Here's how the part is built. I have some questions about the finished solid (model axes, mm). Face numbers are marked on the shaded views. A direction names the side the tool comes from. Coordinates: 2 decimals unless noted, no trailing zeros. Order: outer loops, then holes, each group sorted by start corner. A loop starts at its lowest first (then second) coordinate and runs counter-clockwise, first axis right, second up. Notation, with made-up numbers: (21, 39) - (28, 39) arc R32 ccw to (28, 67) - close; hole circle Ø8 at (-2.5, 13.5). An arc over 180 degrees is marked (long way). Answer as CSV lines item,"result". Start each with the question number.
Q1. I need wall thicknesses on line 1 (X direction, y = -12, z = 24.5); line 2 (X direction, y = 99, z = 22); line 3 (Y direction, x = -56, z = 25). Which ranges of each line are inside material? Lowest first, please.
Q2. Suppose I cut it at D-D (x = 5.5). Please give me the cut outline in (y, z).
Q3. For pin 1 Ø2 at (x, y) = (26, 102.5) entering from +Z; pin 2 Ø12.5 at (y, z) = (105.5, 34.5) entering from +X; pin 3 Ø7.5 at (x, z) = (46, 32) entering from +Y, each with a flat end and sliding along its axis, tell me the tip position at first contact or that it passes through.
Q4. For the marked faces 1, 2 and 3, which set-ups out of +Z, -Z, +X, -X, +Y, -Y let a thin tool reach every point of the face, with its end or its side?
Q5. Suppose I cut it at B-B (y = 43.5). Please give me the cut outline in (x, z).
Q6. Suppose I cut it at C-C (z = 21). Please give me the cut outline in (x, y).
Q7. Thinking about a two-plate mould opening in X: for the marked faces 4, 5 and 6, which applies, released by +X, released by -X, zero draft, split by the parting line, or undercut?
Q8. Suppose I cut it at A-A (z = 37). Please give me the cut outline in (x, y), then the cut area to 3 significant figures.
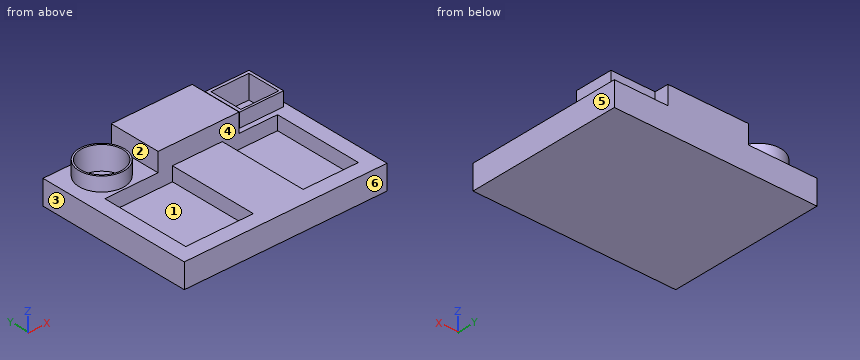
from build123d import *

# Parameters (mm, degrees)
F0_W      = 216
F0_H      = 166
F1_DEPTH  = 26
F2_W      = 184
F2_H      = 95
F3_DEPTH  = 15
F4_W      = 86.176178
F4_H      = 55
F5_DEPTH  = 20
F6_W      = 53.007906
F6_H      = 95
F7_DEPTH  = 15
F8_R      = 24.127346
F9_DEPTH  = 15
F10_R     = 22.341692
F11_DEPTH = 25
F12_W     = 46.807702
F12_H     = 40.58332
F13_DEPTH = 15
F14_W     = 40.349298
F14_H     = 35.074882
F15_DEPTH = 25


with BuildPart() as f1:
    # F0 (on Top) → F1 (new body)
    with BuildSketch(Plane.XY):
        with Locations((-35.592673, 44.704702)):
            Rectangle(F0_W, F0_H)
    extrude(amount=F1_DEPTH)

    # F2 (on face) → F3 (cut)
    with BuildSketch(Plane.XY.offset(26)):
        with Locations((-35.592673, 25.204702)):
            Rectangle(F2_W, F2_H)
    extrude(amount=-F3_DEPTH, mode=Mode.SUBTRACT)

    # F4 (on face) → F5 (join)
    with BuildSketch(Plane.XY.offset(26)):
        with Locations((-27.75256, 100.204702)):
            Rectangle(F4_W, F4_H)
    extrude(amount=F5_DEPTH)

    # F6 (on face) → F7 (join)
    with BuildSketch(Plane.XY.offset(11)):
        with Locations((-28.99965, 25.204702)):
            Rectangle(F6_W, F6_H)
    extrude(amount=F7_DEPTH)

    # F8 (on face) → F9 (join)
    with BuildSketch(Plane.XY.offset(26)):
        with Locations((-106.665462, 99.426791)):
            Circle(F8_R)
    extrude(amount=F9_DEPTH)

    # F10 (on face) → F11 (cut)
    with BuildSketch(Plane.XY.offset(41)):
        with Locations((-106.665462, 99.426791)):
            Circle(F10_R)
    extrude(amount=-F11_DEPTH, mode=Mode.SUBTRACT)

    # F12 (on face) → F13 (join)
    with BuildSketch(Plane.XY.offset(26)):
        with Locations((44.370124, 98.360058)):
            Rectangle(F12_W, F12_H)
    extrude(amount=F13_DEPTH)

    # F14 (on face) → F15 (cut)
    with BuildSketch(Plane.XY.offset(41)):
        with Locations((44.578489, 97.976323)):
            Rectangle(F14_W, F14_H)
    extrude(amount=-F15_DEPTH, mode=Mode.SUBTRACT)


solid = f1.part
Here are the results:
1,line 1,"x = -143.59 to -127.59, -55.5 to -2.5, 56.41 to 72.41"
1,line 2,"x = -143.59 to -129, -84.33 to 24.4, 64.75 to 72.41"
1,line 3,"y = -38.3 to -22.3, 72.7 to 127.7"
2,outline,"(-38.3, 0) - (127.7, 0) - (127.7, 46) - (72.7, 46) - (72.7, 11) - (-22.3, 11) - (-22.3, 26) - (-38.3, 26) - close"
3,pin 1,"stops at z = 16"
3,pin 2,"stops at x = 67.77"
3,pin 3,"stops at y = 118.65"
4,face 1,"+Z"
4,face 2,"+Z, +Y, -Y"
4,face 3,"+Z, -Z, -X, +Y, -Y"
5,outline,"(-143.59, 0) - (72.41, 0) - (72.41, 26) - (56.41, 26) - (56.41, 11) - (-2.5, 11) - (-2.5, 26) - (-55.5, 26) - (-55.5, 11) - (-127.59, 11) - (-127.59, 26) - (-143.59, 26) - close"
6,outline,"(-143.59, -38.3) - (72.41, -38.3) - (72.41, 127.7) - (-143.59, 127.7) - close; hole circle Ø44.68 at (-106.67, 99.43); hole (-127.59, -22.3) - (-55.5, -22.3) - (-55.5, 72.7) - (-127.59, 72.7) - close; hole (-2.5, -22.3) - (56.41, -22.3) - (56.41, 72.7) - (-2.5, 72.7) - close; hole (24.4, 80.44) - (64.75, 80.44) - (64.75, 115.51) - (24.4, 115.51) - close"
7,face 4,"undercut"
7,face 5,"released by +X"
7,face 6,"zero draft"
8,outline,"circle Ø48.25 at (-106.67, 99.43); (-70.84, 72.7) - (15.34, 72.7) - (15.34, 127.7) - (-70.84, 127.7) - close; (20.97, 78.07) - (67.77, 78.07) - (67.77, 118.65) - (20.97, 118.65) - close; hole circle Ø44.68 at (-106.67, 99.43); hole (24.4, 80.44) - (64.75, 80.44) - (64.75, 115.51) - (24.4, 115.51) - close"
8,area,"5,480 mm²"
